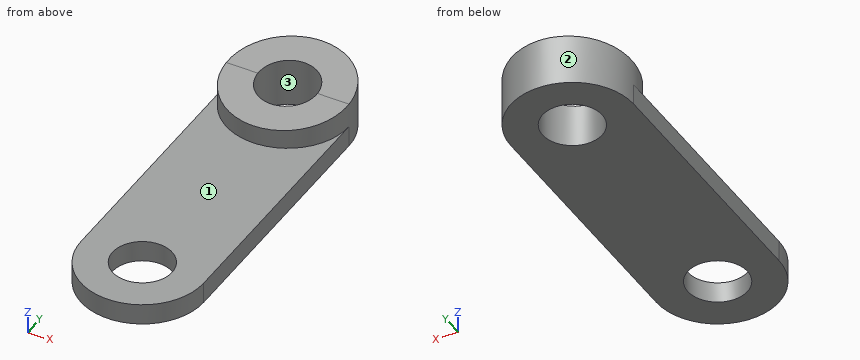
Autodesk Inventor part; units mm, degrees
ref_plane "YZ Plane" through (0, 0, 0) normal (1, 0, 0) x (0, 1, 0)
ref_plane "XZ Plane" through (0, 0, 0) normal (0, 1, 0) x (-1, 0, 0)
ref_plane "XY Plane" through (0, 0, 0) normal (0, 0, 1) x (1, 0, 0)
sketch "Náčrt1" plane through (0, 0, 0) normal (0, 0, 1) x (1, 0, 0)
  line L0 (0, 7.375) -> (0, -7.375) construction
  line L1 (-3.5, 7.375) -> (-3.5, -7.375)
  line L2 (3.5, -7.375) -> (3.5, 7.375)
  arc A0 (3.5, 7.375) -> (-3.5, 7.375) centre (0, 7.375) ccw
  arc A1 (-3.5, -7.375) -> (3.5, -7.375) centre (0, -7.375) ccw
  circle A2 centre (0, 7.375) radius 1.7
  circle A3 centre (0, -7.375) radius 1.7
  circle A4 centre (0, 7.375) radius 3.5
  point P0 (0, 0)
  point P1 (0, 0)
  point P2 (-3.5, 7.375)
  point P3 (3.5, 7.375)
  dimension "d0" = 14.75
  dimension "d1" = 3.5
  dimension "d2" = 3.4
extrude "Vysunutí1" add sketch "Náčrt1" along normal blind 1.2
extrude "Vysunutí2" add sketch "Náčrt1" along normal blind 2.6 contours A0 A4
sketch "Náčrt4" plane through (3.5, -7.375, 0) normal (1, 0, 0) x (0, 0, -1)
  line L0 (-2.6, 13.05) -> (-2.6, 16.45)
  line L1 (-1.2, -1.7) -> (-1.2, 1.7)
  line L2 (-2.6, 14.75) -> (-1.2, 0)
  line L3 (-2.6, 18.25) -> (-2.6, 11.25)
  line L4 (0, 14.75) -> (0, 14.75)
  line L5 (0, 14.75) -> (-1.2, 14.75)
  line L6 (-1.2, 14.75) -> (-1.2, 14.75)
  line L7 (0, 14.75) -> (-1.2, 14.75)
  line L8 (-1.2, 11.25) -> (-2.6, 11.25)
  line L9 (-2.6, 14.75) -> (-2.9322, 18.25)
  line L10 (-2.6, 18.25) -> (-2.9322, 18.25)
  point P0 (0, 7.375)
  point P1 (-2.2678, 11.25)
extrude "Vysunutí3" cut sketch "Náčrt4" against normal through all contours L0 L2 L8 L3
extrude "Vysunutí4" add sketch "Náčrt4" against normal up to surface (7 mm away) contours L9 L10 L3 L0
sketch "Náčrt5" plane through (0, 0, 0) normal (0, 0, -1) x (-1, 0, 0)
  circle A0 centre (0, 7.375) radius 1.7
  circle A1 centre (0, -7.375) radius 1.7
  line L0 (-3.5, -7.375) -> (-3.5, 7.375)
  arc A2 (-3.5, -7.375) -> (3.5, -7.375) centre (0, -7.375) ccw
  line L1 (3.5, 7.375) -> (3.5, -7.375)
  arc A3 (3.5, 7.375) -> (-3.5, 7.375) centre (0, 7.375) ccw
  arc A4 (1.7, 7.375) -> (-1.7, 7.375) centre (0, 7.375) ccw
  line L2 (-1.7, 7.375) -> (1.7, 7.375)
  arc A5 (3.5, 7.375) -> (0, 10.875) centre (0, 7.375) ccw
  line L3 (3.5, 10.875) -> (3.5, 7.375)
  line L4 (0, 10.875) -> (3.5, 10.875)
  arc A6 (0, 10.875) -> (-3.5, 7.375) centre (0, 7.375) ccw
  line L5 (-3.5, 10.875) -> (0, 10.875)
  line L6 (-3.5, 7.375) -> (-3.5, 10.875)
  point P0 (0, 0)
  point P1 (3.5, 7.375)
  point P2 (0, 10.875)
  point P3 (0, 10.875)
  point P4 (-3.5, 7.375)
  point P5 (-1.7, 7.375)
extrude "Vysunutí5" cut sketch "Náčrt5" against normal through all contours L2 A0 | L6 L5 A3 | L4 L3 A3 picked at (0.5018, 7.6383)
properties part number "back qre flex holder"
Part model, mm, in its own coordinate system. Face numbers are marked on the shaded views. Round coordinates to 2 decimals unless told otherwise and drop trailing zeros. Loops run counter-clockwise (first coordinate to the right, second up) from the corner with the lowest first, then second, coordinate; pieces in that order, holes last. Notation, with made-up numbers: (26, 0.5) -> (80, 0.5) arc R35 ccw to (80, 33.5) -> close; hole circle Ø2 at (-1, -17.5). An arc over 180 degrees is marked (long way). Use CSV: the item, a comma, the result in double quotes. Start each with the question number.
1) Cut at D-D, the plane x = 1.5. Write the cut outline in (y, z) (3 decimals), plus the area to 3 significant figures.
2) Cut at A-A, the plane x = 0. Write the cut outline in (y, z) (3 decimals).
3) Drop flat-ended pins along their axis: P1, Ø1, axis at x = -1.5, z = 2.5, coming from the +Y side; P2, Ø2.5, axis at x = 0, y = 7.375, coming from the +Z side; P3, Ø2, axis at x = -2.5, y = -6, coming from the +Z side. Give the stop position or say it passes through.
4) Cut at B-B, the plane z = 0.4. Write the cut outline in (x, y) (3 decimals).
5) Pull direction X, two halves, no side cores. Call the marked faces 1, 2 and 3: +X half, -X half, draft (parallel to the pull), parting line (faces both ways), or undercut.
6) Cut at C-C, the plane y = 8.25. Write the cut outline in (x, z), plus the area to 3 significant figures.
7) Wall check: L1, parallel to Y at x = 0, z = 0.9 (3 decimals); L2, parallel to Y at x = 1.5, z = 0.7 (3 decimals); L3, parallel to X at y = -7.25, z = 1. Give the ranges that are in metal, low to high. Write a range as [from, to].
Determined:
1,outline,"(-10.537, 0) -> (-8.175, 0) -> (-8.175, 1.2) -> (-10.537, 1.2) -> close; (-6.575, 0) -> (6.575, 0) -> (6.575, 2.524) -> (4.213, 2.3) -> (4.213, 1.2) -> (-6.575, 1.2) -> close; (8.175, 0) -> (10.537, 0) -> (10.537, 2.9) -> (8.175, 2.676) -> close"
1,area,"28.1 mm2"
2,outline,"(-10.875, 0) -> (-9.075, 0) -> (-9.075, 1.2) -> (-10.875, 1.2) -> close; (-5.675, 0) -> (5.675, 0) -> (5.675, 2.439) -> (3.875, 2.268) -> (3.875, 1.2) -> (-5.675, 1.2) -> close; (9.075, 0) -> (10.875, 0) -> (10.875, 2.932) -> (9.075, 2.761) -> close"
3,P1,"stops at y = 10.73"
3,P2,"passes through"
3,P3,"stops at z = 1.2"
4,outline,"(-3.5, -7.375) arc R3.5 ccw to (3.5, -7.375) -> (3.5, 7.375) arc R3.5 ccw to (-3.5, 7.375) -> close; hole circle Ø3.4 at (0, -7.375); hole circle Ø3.4 at (0, 7.375)"
5,face 1,"draft"
5,face 2,"parting line"
5,face 3,"undercut"
6,outline,"(-3.39, 0) -> (-1.46, 0) -> (-1.46, 2.68) -> (-3.39, 2.68) -> close; (1.46, 0) -> (3.39, 0) -> (3.39, 2.68) -> (1.46, 2.68) -> close"
6,area,"10.4 mm2"
7,L1,"y = [-10.875, -9.075], [-5.675, 5.675], [9.075, 10.875]"
7,L2,"y = [-10.537, -8.175], [-6.575, 6.575], [8.175, 10.537]"
7,L3,"x = [-3.5, -1.7], [1.7, 3.5]"
